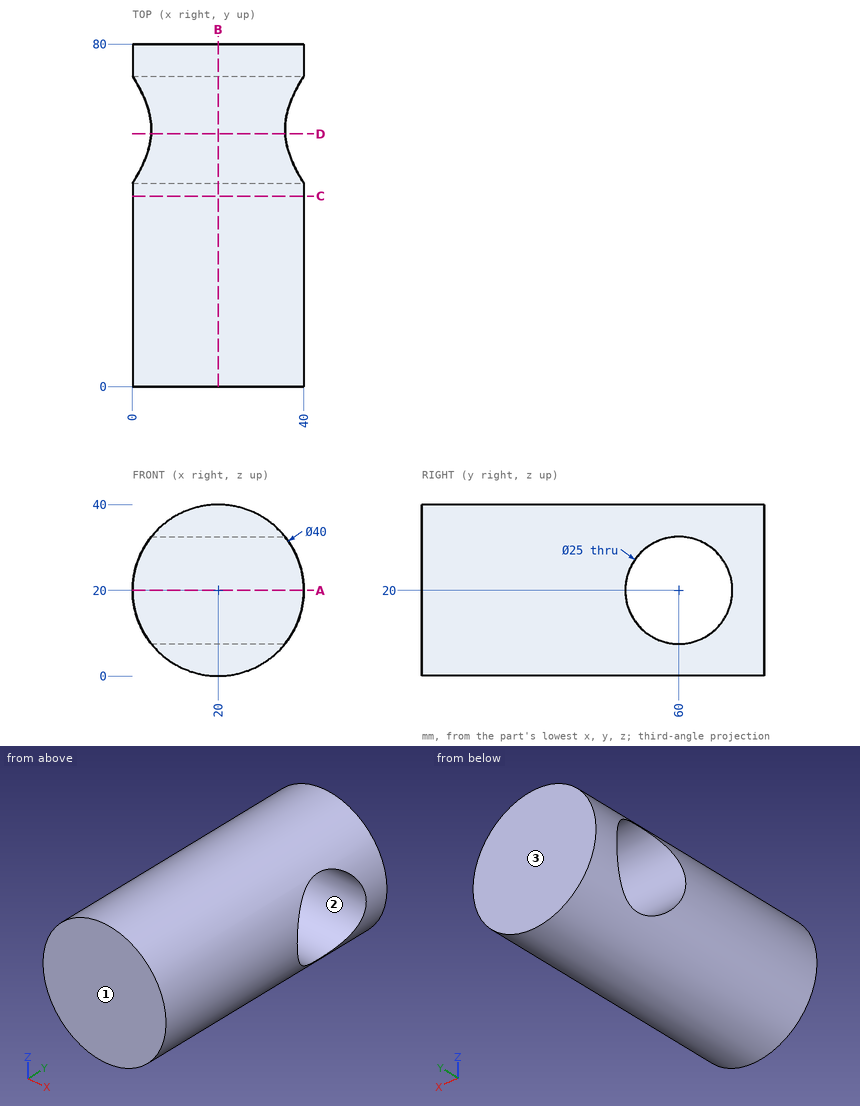
Study the drawing (mm; zero at the part's minimum x, y, z) and answer. Round coordinates to 2 decimals unless told otherwise and drop trailing zeros. Write each loop counter-clockwise with the first axis right and the second up, starting at its lowest first coordinate (ties: lowest second). Pieces come first, ordered by that corner, then holes. Notation, with made-up numbers: (69, -10.75) -> (74, -10.75) arc R21 cw to (74, -3.75) -> close; hole circle Ø3 at (34.25, 14.25). An arc over 180 degrees is marked (long way). Write item = value, one per line.
1) Section C-C on y = 44.5 is taken. Write down the section's boundary in (x, z).
Check values:
outline = circle Ø40 at (20, 20)
2) Section B-B on x = 20 is taken. Write down the section's boundary in (y, z).
Check values:
outline = (0, 0) -> (80, 0) -> (80, 40) -> (0, 40) -> close; hole circle Ø25 at (60, 20)
3) For a pull along Y with two mould halves and no side action, classify the marked faces 1, 2 and 3 as released by +Y, released by -Y, zero draft, split by the parting line, or undercut.
Check values:
face_1 = released by -Y
face_2 = undercut
face_3 = released by +Y
4) Section D-D on y = 59 is taken. Write down the section's boundary in (x, z), plus the area to 3 significant figures.
Check values:
outline = (4.36, 7.54) arc R20 ccw to (35.64, 7.54) -> close; (4.36, 32.46) -> (35.64, 32.46) arc R20 ccw to start
area = 329 mm²
5) Section A-A on z = 20 is taken. Write down the section's boundary in (x, y).
Check values:
outline = (0, 0) -> (40, 0) -> (40, 47.5) -> (0, 47.5) -> close; (0, 72.5) -> (40, 72.5) -> (40, 80) -> (0, 80) -> close
6) Straight lines are drawn through the part: line 1 along Y through (x, z) = (16, 19.5); line 2 along Z through (x, y) = (13, 65) (3 decimals); line 3 along Z through (x, y) = (29, 56). For each, find the intervals that lie inside material, in ascending order. Write a range as [from, to].
Check values:
line_1 = [0, 47.51], [72.49, 80]
line_2 = [1.265, 8.544], [31.456, 38.735]
line_3 = [2.14, 8.16], [31.84, 37.86]
7) Given pin 1 (1.5 mm diameter, centred on y = 24.5, z = 10, fed in from +X); pin 2 (5 mm diameter, centred on x = 7.5, z = 4, fed in from -Y); pin 3 (6 mm diameter, centred on y = 21, z = 14.5, fed in from +X); pin 4 (10 mm diameter, centred on x = 18.5, y = 60, fed in from -Z), each flat-ended and moving along its own axis, determine where each tip first touches the part or whether it passes through.
Check values:
pin_1 = 37.73
pin_2 = 0
pin_3 = 39.84
pin_4 = 0
